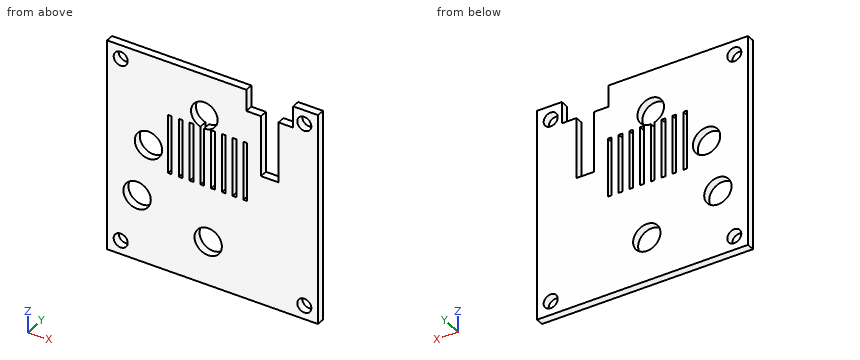
```python
from build123d import *

# Parameters (mm, degrees)
SKETCH_3_R      = 3.5
SKETCH_3_W      = 0.91875
SKETCH_3_H      = 15
SKETCH_3_R_2    = 1.8
EXTRUDE_2_DEPTH = 2


with BuildPart() as part:
    # 草图3 → 凸台-拉伸2 (new body)
    with BuildSketch(Plane(origin=(0, 0, 0), x_dir=(1, 0, 0), z_dir=(0, 1, 0))):
        Polygon((16.9, -21.5), (20.65, -21.5), (20.65, -27), (27, -27), (27, 27), (-27, 27), (-27, -27), (8.65, -27), (8.65, -21.5), (12.4, -21.5), (12.4, -6), (16.9, -6), align=None)
        with Locations((-19.3, 10.3)):
            Circle(SKETCH_3_R, mode=Mode.SUBTRACT)
        with Locations((-16.4, -3.7)):
            Circle(SKETCH_3_R, mode=Mode.SUBTRACT)
        with Locations((-10.896875, -5.8)):
            Rectangle(SKETCH_3_W, SKETCH_3_H, mode=Mode.SUBTRACT)
        with BuildLine():
            Line((-3.0875, -13.246564316), (-3.0875, 1.7))
            Line((-3.0875, 1.7), (-2.16875, 1.7))
            Line((-2.16875, 1.7), (-2.16875, -13.100695154))
            ThreePointArc((-2.16875, -13.100695154), (-1.566862617, -19.857940519), (-3.0875, -13.246564316))
        make_face(mode=Mode.SUBTRACT)
        with Locations((-8.140625, -5.8)):
            Rectangle(SKETCH_3_W, SKETCH_3_H, mode=Mode.SUBTRACT)
        with Locations((-5.384375, -5.8)):
            Rectangle(SKETCH_3_W, SKETCH_3_H, mode=Mode.SUBTRACT)
        with Locations((0.128125, -5.8)):
            Rectangle(SKETCH_3_W, SKETCH_3_H, mode=Mode.SUBTRACT)
        with Locations((23.5, -23.5)):
            Circle(SKETCH_3_R_2, mode=Mode.SUBTRACT)
        with Locations((2.884375, -5.8)):
            Rectangle(SKETCH_3_W, SKETCH_3_H, mode=Mode.SUBTRACT)
        with Locations((5.640625, -5.8)):
            Rectangle(SKETCH_3_W, SKETCH_3_H, mode=Mode.SUBTRACT)
        with Locations((8.396875, -5.8)):
            Rectangle(SKETCH_3_W, SKETCH_3_H, mode=Mode.SUBTRACT)
        with Locations((-1.1, 15.8)):
            Circle(SKETCH_3_R, mode=Mode.SUBTRACT)
        with Locations((23.5, 23.5)):
            Circle(SKETCH_3_R_2, mode=Mode.SUBTRACT)
        with Locations((-23.5, -23.5)):
            Circle(SKETCH_3_R_2, mode=Mode.SUBTRACT)
        with Locations((-23.5, 23.5)):
            Circle(SKETCH_3_R_2, mode=Mode.SUBTRACT)
    extrude(amount=EXTRUDE_2_DEPTH)


solid = part.part
```
Input: part model. Units: mm. Frame: model coordinates. Round coordinates to 2 decimals unless told otherwise and drop trailing zeros. Loops run counter-clockwise (first coordinate to the right, second up) from the corner with the lowest first, then second, coordinate; pieces in that order, holes last. Notation, with made-up numbers: (-25, 52) -> (2, 52) arc R27 ccw to (2, 85) -> close; hole circle Ø2 at (3, 2.25). An arc over 180 degrees is marked (long way). One line per item, written item: value.
(1) Pin query (flat end, axial travel): pin 1 (10 mm diameter, centred on x = -9, z = -18.5, fed in from -Y); pin 2 (1 mm diameter, centred on x = 18, y = 0.5, fed in from +Z). Return the tip coordinate at first contact, or that it passes through.
Geometry check:
pin 1: y = 0
pin 2: z = 21.5
(2) Section C-C (x = -23.5). Return the cut outline in (y, z), plus the area to 3 significant figures.
Geometry check:
outline: (0, -27) -> (2, -27) -> (2, -25.3) -> (0, -25.3) -> close; (0, -21.7) -> (2, -21.7) -> (2, 21.7) -> (0, 21.7) -> close; (0, 25.3) -> (2, 25.3) -> (2, 27) -> (0, 27) -> close
area: 93.6 mm2
(3) Section A-A (z = -15.8). Return the cut outline in (x, y), plus the area to 3 significant figures.
Geometry check:
outline: (-27, 0) -> (-4.6, 0) -> (-4.6, 2) -> (-27, 2) -> close; (2.4, 0) -> (27, 0) -> (27, 2) -> (2.4, 2) -> close
area: 94.0 mm2
(4) Material intervals for line 1 (Z direction, x = -23.5, y = 0.65); line 2 (X direction, y = 1.3, z = 23.5); line 3 (Z direction, x = -19.3, y = 1.15), sorted ascending. Write a range as [from, to].
Geometry check:
line 1: [-27, -25.3], [-21.7, 21.7], [25.3, 27]
line 2: [-27, -25.3], [-21.7, 8.65], [20.65, 21.7], [25.3, 27]
line 3: [-27, -13.8], [-6.8, 1.74], [5.66, 27]
(5) Section D-D (z = 16.5). Return the cut outline in (x, y).
Geometry check:
outline: (-27, 0) -> (-5.5, 0) -> (-5.5, 2) -> (-27, 2) -> close; (1.3, 0) -> (12.4, 0) -> (12.4, 2) -> (1.3, 2) -> close; (16.9, 0) -> (27, 0) -> (27, 2) -> (16.9, 2) -> close
(6) Section B-B (z = 23.5). Return the cut outline in (x, y).
Geometry check:
outline: (-27, 0) -> (-25.3, 0) -> (-25.3, 2) -> (-27, 2) -> close; (-21.7, 0) -> (8.65, 0) -> (8.65, 2) -> (-21.7, 2) -> close; (20.65, 0) -> (21.7, 0) -> (21.7, 2) -> (20.65, 2) -> close; (25.3, 0) -> (27, 0) -> (27, 2) -> (25.3, 2) -> close
